Verification items for the finished model (mm, model axes). A direction names the side the tool comes from. Give positions to 0.01 mm unless a question says otherwise; leave off trailing zeros. Order: outer loops, then holes, each group sorted by start corner. A loop starts at its lowest first (then second) coordinate and runs counter-clockwise, first axis right, second up. Notation, with made-up numbers: (50, 5) - (93, 5) arc R11 ccw to (93, 14) - close; hole circle Ø8 at (-25.75, 82). An arc over 180 degrees is marked (long way). Answer as a JSON object with one key per item and string values. Group by question number.
(1) Section check B-B (x = -8.5). Record the boundary of the cut face in (y, z), then the cut area to 3 significant figures.
(2) Section check C-C (y = 1.4). Record the boundary of the cut face in (x, z) (3 decimals).
(3) Thickness scan on line 1 (X direction, y = 1.6, z = 13); line 2 (X direction, y = 0.95, z = -7.5); line 3 (Z direction, x = 4, y = 0.9). Record the ranges inside material, lowest first.
(4) Section check D-D (z = 15.5). Record the boundary of the cut face in (x, y).
(5) Mould release check, pull along Z, two halves, no side actions. Record for faces 1 (the face through (11, 1.75, 0)), 2 (the face through (7.204, 0.887, -13.97)), 3 (the face through (-0.405, 0.863, -25.457)), 4 (the face through (-6.12, 0.89, -5.9)): +Z half, -Z half, draft (parallel to the pull), parting line (faces both ways), or undercut.
(6) Section check A-A (x = 0). Record the boundary of the cut face in (y, z).
(7) Access from +Z, -Z, +X, -X, +Y, -Y to the whole of each face (thin tool, end or side, straight path). Record for faces 5 (the face through (1.891, 0.863, 10.653)), 6 (the face through (11, 0, 0)).
```python
from build123d import *

# Parameters (mm, degrees)
BOSS_EXTRUDE1_DEPTH = 1.75
CUT_EXTRUDE1_DEPTH  = 2.75
CUT_EXTRUDE2_DEPTH  = 1.75
FILLET2_R           = 5
FILLET1_R           = 4
SKETCH6_R           = 1.25
CUT_EXTRUDE3_DEPTH  = 2.75
CIRPATTERN3_COUNT   = 2


with BuildPart() as part:
    # Sketch1 → Boss-Extrude1 (new body)
    with BuildSketch(Plane(origin=(0, 0, 0), x_dir=(1, 0, 0), z_dir=(0, 1, 0))):
        with BuildLine():
            Line((-23.1, -10.705213683), (-23.1, 10.705213683))
            ThreePointArc((-23.1, 10.705213683), (0, 25.46), (23.1, 10.705213683))
            Line((23.1, 10.705213683), (23.1, -10.705213683))
            ThreePointArc((23.1, -10.705213683), (0, -25.46), (-23.1, -10.705213683))
        make_face()
    extrude(amount=BOSS_EXTRUDE1_DEPTH)

    # Sketch3 → Cut-Extrude1 (cut, through all)
    with BuildSketch(Plane(origin=(0, 1.75, 0), x_dir=(1, 0, 0), z_dir=(0, 1, 0))):
        Polygon((0, -12.02081528), (-12.02081528, 0), (0, 12.02081528), (12.02081528, 0), align=None)
    extrude(amount=-CUT_EXTRUDE1_DEPTH, mode=Mode.SUBTRACT)

    # Sketch4 → Cut-Extrude2 (cut)
    with BuildSketch(Plane(origin=(0, 1.75, 0), x_dir=(1, 0, 0), z_dir=(0, 1, 0))):
        with BuildLine():
            Line((-1.5, 13), (-1.5, -13))
            ThreePointArc((-1.5, -13), (0, -14.5), (1.5, -13))
            Line((1.5, -13), (1.5, 13))
            ThreePointArc((1.5, 13), (0, 14.5), (-1.5, 13))
        make_face()
    extrude(amount=-CUT_EXTRUDE2_DEPTH, mode=Mode.SUBTRACT)

    # Fillet2
    fillet2_edges = [part.edges().sort_by_distance(p)[0] for p in [
        (1.5, 0.875, -10.52081528),
        (-1.5, 0.875, -10.52081528),
        (-1.5, 0.875, 10.52081528),
        (1.5, 0.875, 10.52081528),
    ]]
    fillet(fillet2_edges, radius=FILLET2_R)

    # Fillet1
    fillet1_edges = [part.edges().sort_by_distance(p)[0] for p in [
        (12.02081528, 0.875, 0),
        (-12.02081528, 0.875, 0),
    ]]
    fillet(fillet1_edges, radius=FILLET1_R)

    # Sketch6 → Cut-Extrude3 (cut, through all)
    with BuildSketch(Plane(origin=(0, 1.75, 0), x_dir=(1, 0, 0), z_dir=(0, 1, 0))):
        with Locations((-8.125, 13.125)):
            Circle(SKETCH6_R)
        with Locations((8.125, 13.125)):
            Circle(SKETCH6_R)
    cut_extrude3 = extrude(amount=-CUT_EXTRUDE3_DEPTH, mode=Mode.SUBTRACT)

    # CirPattern3: Cut-Extrude3 ×2 about axis
    cirpattern3_axis = Axis((0, 0, 0), (0, 1, 0))
    for i in range(1, CIRPATTERN3_COUNT):
        add(cut_extrude3.rotate(cirpattern3_axis, i * 360 / CIRPATTERN3_COUNT), mode=Mode.SUBTRACT)


solid = part.part
```
Solutions:
{
 "1": {"outline": "(0, -24) - (1.75, -24) - (1.75, -14.32) - (0, -14.32) - close; (0, -11.93) - (1.75, -11.93) - (1.75, -3.52) - (0, -3.52) - close; (0, 3.52) - (1.75, 3.52) - (1.75, 11.93) - (0, 11.93) - close; (0, 14.32) - (1.75, 14.32) - (1.75, 24) - (0, 24) - close", "area": "63.3 mm2"},
 "2": {"outline": "(-23.1, -10.705) arc R25.46 ccw to (23.1, -10.705) - (23.1, 10.705) arc R25.46 ccw to (-23.1, 10.705) - close; hole circle Ø2.5 at (-8.125, -13.125); hole circle Ø2.5 at (-8.125, 13.125); hole (-9.192, -2.828) - (-2.964, -9.056) arc R5 cw to (-1.5, -12.592) - (-1.5, -13) arc R1.5 ccw to (1.5, -13) - (1.5, -12.592) arc R5 cw to (2.964, -9.056) - (9.192, -2.828) arc R4 ccw to (9.192, 2.828) - (2.964, 9.056) arc R5 cw to (1.5, 12.592) - (1.5, 13) arc R1.5 ccw to (-1.5, 13) - (-1.5, 12.592) arc R5 cw to (-2.964, 9.056) - (-9.192, 2.828) arc R4 ccw to start; hole circle Ø2.5 at (8.125, -13.125); hole circle Ø2.5 at (8.125, 13.125)"},
 "3": {"line 1": "x = -21.89 to -9.37, -6.88 to -1.5, 1.5 to 6.88, 9.37 to 21.89", "line 2": "x = -23.1 to -4.52, 4.52 to 23.1", "line 3": "z = -25.14 to -8.02, 8.02 to 25.14"},
 "4": {"outline": "(-20.2, 0) - (20.2, 0) - (20.2, 1.75) - (-20.2, 1.75) - close"},
 "5": {"face 1": "draft", "face 2": "undercut", "face 3": "-Z half", "face 4": "undercut"},
 "6": {"outline": "(0, -25.46) - (1.75, -25.46) - (1.75, -14.5) - (0, -14.5) - close; (0, 14.5) - (1.75, 14.5) - (1.75, 25.46) - (0, 25.46) - close"},
 "7": {"face 5": "+Y, -Y", "face 6": "+Z, -Z, +X, -X, -Y"}
}
